Can you work these out from the model? Positions are in its coordinate system, mm. A direction names the side the tool comes from. Give positions to 0.01 mm unless a question says otherwise; leave off trailing zeros. Order: outer loops, then holes, each group sorted by start corner. A loop starts at its lowest first (then second) coordinate and runs counter-clockwise, first axis right, second up. Notation, with made-up numbers: (-29, -12.5) - (24, -12.5) arc R14 cw to (24, -8.5) - close; hole circle Ø6 at (85.25, 0.25). An arc over 180 degrees is marked (long way). Answer as CSV lines item,"result".
```python
from build123d import *

# Parameters (mm, degrees)
F2_SIZE2 = 2
F2_SIZE  = 2
F4_DEPTH = 100


with BuildPart() as f1:
    # F0 (on Top) → F1 (revolve)
    with BuildSketch(Plane.XY):
        Polygon((0, 80), (0, 0), (21, 0), (21, 25), (14, 25), (14, 40), (9, 40), (9, 43), (11, 43), (11, 80), align=None)
    revolve(axis=Axis((0, 40, 0), (0, -1, 0)))

    # F2
    f2_edges = [f1.edges().sort_by_distance(p)[0] for p in [
        (-11, 80, 0),
        (-21, 0, 0),
    ]]
    chamfer(f2_edges, length=F2_SIZE, length2=F2_SIZE2)

    # F3 (on Front) → F4 (cut)
    with BuildSketch(Plane.XZ):
        with BuildLine():
            Line((-7.75, 3.584375), (7.75, 3.584375))
            ThreePointArc((7.75, 3.584375), (0, 8.53875), (-7.75, 3.584375))
        make_face()
        with BuildLine():
            ThreePointArc((-7.75, -3.584375), (0, -8.53875), (7.75, -3.584375))
            Line((7.75, -3.584375), (-7.75, -3.584375))
        make_face()
    extrude(amount=-F4_DEPTH, mode=Mode.SUBTRACT)


solid = f1.part
```
1) I need wall thicknesses on line 1 along Z through (x, y) = (-5.5, 53); line 2 along Y through (x, z) = (-8.5, -14.5); line 3 along Z through (x, y) = (6, 23.5). Which ranges of each line are inside material? Lowest first, please. Write a range as [from, to].
Answer block:
line 1,"[-9.53, -6.53], [-3.58, 3.58], [6.53, 9.53]"
line 2,"[0, 25]"
line 3,"[-20.12, -6.08], [-3.58, 3.58], [6.08, 20.12]"
2) Which directions (+Z, -Z, +X, -X, +Y, -Y) give clear straight access to the entire face, cutting with the end or side of a thin tool? Please do faces 1 (the flat face through (9, 40, -3)), 2 (the cylindrical face through (-2.38, 60.74, -10.74)), 3 (the flat face through (0, 39, -3.584)), 4 (the flat face through (0, 0, 0)).
Answer block:
face 1,"none"
face 2,"+Y"
face 3,"+Y, -Y"
face 4,"+Z, -Z, +X, -X, -Y"
3) I want a section at D-D on y = 41.5. Write out the boundary of the cut face in (x, z), plus the area to 3 significant figures.
Answer block:
outline,"circle Ø18 at (0, 0); hole (-7.75, -3.58) arc R8.54 ccw to (7.75, -3.58) - close; hole (-7.75, 3.58) - (7.75, 3.58) arc R8.54 ccw to start"
area,"144 mm2"
4) I want a section at A-A on x = 0. Write out the boundary of the cut face in (y, z).
Answer block:
outline,"(0, -19) - (2, -21) - (25, -21) - (25, -14) - (40, -14) - (40, -9) - (43, -9) - (43, -11) - (78, -11) - (80, -9) - (80, -8.54) - (0, -8.54) - close; (0, -3.58) - (80, -3.58) - (80, 3.58) - (0, 3.58) - close; (0, 8.54) - (80, 8.54) - (80, 9) - (78, 11) - (43, 11) - (43, 9) - (40, 9) - (40, 14) - (25, 14) - (25, 21) - (2, 21) - (0, 19) - close"
5) If we mould it in two halves opening along X, with no side actions, what happens to faces 5 (the flat face through (0, 80, 0)), 6 (the cylindrical face through (12.932, 32.605, -5.362)), 7 (the flat face through (0, 39, 3.584))? For each: +X half, -X half, draft (parallel to the pull), parting line (faces both ways), or undercut.
Answer block:
face 5,"draft"
face 6,"parting line"
face 7,"undercut"
6) I want a section at C-C on z = 0. Write out the boundary of the cut face in (x, y).
Answer block:
outline,"(-21, 2) - (-19, 0) - (19, 0) - (21, 2) - (21, 25) - (14, 25) - (14, 40) - (9, 40) - (9, 43) - (11, 43) - (11, 78) - (9, 80) - (-9, 80) - (-11, 78) - (-11, 43) - (-9, 43) - (-9, 40) - (-14, 40) - (-14, 25) - (-21, 25) - close"
7) I'm going to push flat-ended pins straight in: P1, Ø5, axis at y = 12.5, z = 6, coming from the -X side; P2, Ø1.5, axis at x = -11.5, y = 30.5, coming from the +Z side; P3, Ø12, axis at x = 10.5, y = 50.5, coming from the -Z side. Where does each tip first touch, or does it pass through?
Answer block:
P1,"x = -20.71"
P2,"z = 8.97"
P3,"z = -10.04"
8) I want a section at B-B on y = 51.5. Write out the boundary of the cut face in (x, z).
Answer block:
outline,"circle Ø22 at (0, 0); hole (-7.75, -3.58) arc R8.54 ccw to (7.75, -3.58) - close; hole (-7.75, 3.58) - (7.75, 3.58) arc R8.54 ccw to start"
